```python
from build123d import *

# Parameters (mm, degrees)
F0_R     = 0.6
F1_DEPTH = 2.4
F2_R     = 1


with BuildPart() as f1:
    # F0 (on Top) → F1 (new body)
    with BuildSketch(Plane.XY):
        Polygon((2.5, 8.490209), (2.5, 4.740209), (9, 4.740209), (9, -3.759791), (0, -3.759791), (-9, -3.759791), (-9, 4.740209), (-2.5, 4.740209), (-2.5, 8.490209), (-15, 8.490209), (-15, -7.509791), (0, -7.509791), (15, -7.509791), (15, 8.490209), align=None)
        with Locations((-11, 0)):
            Circle(F0_R, mode=Mode.SUBTRACT)
        with Locations((11, 0)):
            Circle(F0_R, mode=Mode.SUBTRACT)
    extrude(amount=F1_DEPTH)

    # F2
    f2_edges = [f1.edges().sort_by_distance(p)[0] for p in [
        (15, 8.490209, 1.2),
        (15, -7.509791, 1.2),
        (-15, 8.490209, 1.2),
        (-15, -7.509791, 1.2),
    ]]
    fillet(f2_edges, radius=F2_R)


solid = f1.part
```
Source: CAD feature listing. Evaluate the final solid. Frame: model axes, mm. A direction names the side the tool comes from. Round coordinates to 2 decimals unless told otherwise and drop trailing zeros. Loops run counter-clockwise (first coordinate to the right, second up) from the corner with the lowest first, then second, coordinate; pieces in that order, holes last. Notation, with made-up numbers: (5, -23) - (44, -23) arc R20 ccw to (44, -17) - close; hole circle Ø2 at (47, 16.25). An arc over 180 degrees is marked (long way). Use CSV: the item, a comma, the result in double quotes.
Q1. Reachability of faces 4 (the flat face through (-15, 1, 1)), 5 (the flat face through (0, -3.76, 1)), 6 (the flat face through (-2.5, 7, 1)) from +Z, -Z, +X, -X, +Y, -Y: full face, straight path, thin tool, end or side. Return the list, or none.
Reported:
face 4,"+Z, -Z, -X, +Y, -Y"
face 5,"+Z, -Z"
face 6,"+Z, -Z, +Y"
Q2. Ray query, line 1 along Y through (x, z) = (3.25, 1.8); line 2 along Y through (x, z) = (11, 1.6); line 3 along X through (y, z) = (1.5, 0.45). Return the intervals inside material, ascending.
Reported:
line 1,"-7.51 to -3.76, 4.74 to 8.49"
line 2,"-7.51 to -0.6, 0.6 to 8.49"
line 3,"-15 to -9, 9 to 15"
Q3. Pin query (flat end, axial travel): pin 1 Ø5 at (x, y) = (-4.5, 0) entering from -Z; pin 2 Ø5 at (x, y) = (-4.5, -4.5) entering from -Z; pin 3 Ø0.7 at (x, z) = (1, 1.5) entering from +Y. Return the tip coordinate at first contact, or that it passes through.
Reported:
pin 1,"through"
pin 2,"z = 0"
pin 3,"y = -3.76"
Q4. Section query A-A, the plane y = 0. Output: boundary loops of the cut face in (x, z).
Reported:
outline,"(-15, 0) - (-11.6, 0) - (-11.6, 2.4) - (-15, 2.4) - close; (-10.4, 0) - (-9, 0) - (-9, 2.4) - (-10.4, 2.4) - close; (9, 0) - (10.4, 0) - (10.4, 2.4) - (9, 2.4) - close; (11.6, 0) - (15, 0) - (15, 2.4) - (11.6, 2.4) - close"
Q5. Section query D-D, the plane z = 1.65. Output: boundary loops of the cut face in (x, y), then the cut area to 3 significant figures.
Reported:
outline,"(-15, -6.51) arc R1 ccw to (-14, -7.51) - (14, -7.51) arc R1 ccw to (15, -6.51) - (15, 7.49) arc R1 ccw to (14, 8.49) - (2.5, 8.49) - (2.5, 4.74) - (9, 4.74) - (9, -3.76) - (-9, -3.76) - (-9, 4.74) - (-2.5, 4.74) - (-2.5, 8.49) - (-14, 8.49) arc R1 ccw to (-15, 7.49) - close; hole circle Ø1.2 at (-11, 0); hole circle Ø1.2 at (11, 0)"
area,"305 mm^2"
Q6. Section query C-C, the plane y = 3.25. Output: boundary loops of the cut face in (x, z).
Reported:
outline,"(-15, 0) - (-9, 0) - (-9, 2.4) - (-15, 2.4) - close; (9, 0) - (15, 0) - (15, 2.4) - (9, 2.4) - close"
Q7. Section query B-B, the plane x = 4.25. Output: boundary loops of the cut face in (y, z), then the cut area to 3 significant figures.
Reported:
outline,"(-7.51, 0) - (-3.76, 0) - (-3.76, 2.4) - (-7.51, 2.4) - close; (4.74, 0) - (8.49, 0) - (8.49, 2.4) - (4.74, 2.4) - close"
area,"18.0 mm^2"
Q8. Mould query, pull axis Y, two halves, no side actions, for faces 1 (the flat face through (-6, 4.74, 1)), 2 (the flat face through (0, -7.51, 1)), 3 (the flat face through (2.5, 7, 1)). Classes: pulls with the +Y half, pulls with the -Y half, needs draft (parallel to the pull), parting line crosses it, or undercut.
Reported:
face 1,"undercut"
face 2,"pulls with the -Y half"
face 3,"needs draft"
